Could you check a few things on this model? Use its own coordinates, in mm. A direction names the side the tool comes from. Coordinates: 2 decimals unless noted, no trailing zeros. Loops run counter-clockwise (first coordinate to the right, second up) from the corner with the lowest first, then second, coordinate; pieces in that order, holes last.
1) If I drill on line 1 along X through (y, z) = (10.25, -1.75); line 2 along Y through (x, z) = (-3.5, -1.75); line 3 along Y through (x, z) = (4.25, -1.5), over which ranges is the centre line in solid material (lowest first)?
2) Thinking about a two-plate mould opening in Y: for faces 1 (the face through (-2.1, -1.805, -3.3)), 2 (the face through (1.14, 0.17, -4.88)), 3 (the face through (3.65, 8.44, 0.16)), 4 (the face through (2, 2.195, 4)), which applies, released by +Y, released by -Y, zero draft, split by the parting line, or undercut?
3) Imagine slicing it at A-A on z = 0. Please give me the cut outline in (x, y).
4) Imagine slicing it at C-C on y = 1.5. Please give me the cut outline in (x, z).
5) For faces 5 (the face through (3.55, -4.34, 0.15)), 6 (the face through (0.922, 9.829, -3.905)), 7 (the face through (0, -6.805, 0)), which set-ups out of +Z, -Z, +X, -X, +Y, -Y let a thin tool reach every point of the face, with its end or its side?
6) Will these pins go through, and if not, where does the flat tip stop? P1, Ø3, axis at y = 8.5, z = -4, coming from the +X side; P2, Ø3, axis at x = 1.5, y = 4.5, coming from the -Z side; P3, Ø2, axis at y = 4, z = -1.5, coming from the -X side.
7) Imagine slicing it at B-B on y = 7.5. Please give me the cut outline in (x, z), plus the area to 3 significant figures.
8) Imagine slicing it at D-D on z = 4.5. Please give me the cut outline in (x, y), plus the area to 3 significant figures.
```python
from build123d import *

# Parameters (mm, degrees)
FILLET1_R = 0.2


with BuildPart() as part:
    # Sketch2 → Revolve1 (revolve)
    with BuildSketch(Plane.XY):
        Polygon((-3.9451521, 11.195402299), (-3.9451521, 8.695402299), (-3.5451521, 8.695402299), (-3.5451521, 8.195402299), (-3.9451521, 8.195402299), (-3.9451521, 2.195402299), (-4.9451521, 2.195402299), (-4.9451521, -1.804597701), (-3.4451521, -1.804597701), (-3.4451521, -6.804597701), (0.0548479, -6.804597701), (0.0548479, 11.195402299), align=None)
    revolve(axis=Axis((0.0548479, -6.804597701, 0), (0, 1, 0)))

    # Fillet1
    fillet1_edges = [part.edges().sort_by_distance(p)[0] for p in [
        (4.0548479, 11.195402299, 0),
    ]]
    fillet(fillet1_edges, radius=FILLET1_R)


solid = part.part
```
Filled in:
1. line 1: x = -3.54 to 3.65
1. line 2: y = -1.8 to 8.2, 8.7 to 11.11
1. line 3: y = -1.8 to 2.2
2. face 1: released by -Y
2. face 2: zero draft
2. face 3: undercut
2. face 4: released by +Y
3. outline: (-4.95, -1.8) - (-3.45, -1.8) - (-3.45, -6.8) - (3.55, -6.8) - (3.55, -1.8) - (5.05, -1.8) - (5.05, 2.2) - (4.05, 2.2) - (4.05, 8.2) - (3.65, 8.2) - (3.65, 8.7) - (4.05, 8.7) - (4.05, 11) arc R0.2 ccw to (3.85, 11.2) - (-3.75, 11.2) arc R0.2 ccw to (-3.95, 11) - (-3.95, 8.7) - (-3.55, 8.7) - (-3.55, 8.2) - (-3.95, 8.2) - (-3.95, 2.2) - (-4.95, 2.2) - close
4. outline: circle Ø10 at (0.05, 0)
5. face 5: -Y
5. face 6: +Y
5. face 7: +Z, -Z, +X, -X, -Y
6. P1: stops at x = 3.17
6. P2: stops at z = -4
6. P3: stops at x = -3.91
7. outline: circle Ø8 at (0.05, 0)
7. area: 50.3 mm2
8. outline: (-2.12, -1.8) - (2.23, -1.8) - (2.23, 2.2) - (-2.12, 2.2) - close
8. area: 17.4 mm2
